The model under review builds one solid part; all positions refer to its coordinate system, in mm. Coordinates: 2 decimals unless noted, no trailing zeros. Write each loop counter-clockwise with the first axis right and the second up, starting at its lowest first coordinate (ties: lowest second). Pieces come first, ordered by that corner, then holes.
1) For line 1 (Y direction, x = 471, z = -1) (1 decimal); line 2 (Z direction, x = 927.5, y = -10), list the stretches that pass through material, from the lowest coordinate up.
2) For P1, Ø5, axis at y = 5.5, z = -2, coming from the +X side; P2, Ø24.5, axis at x = 553.5, y = 5, coming from the +Z side; P3, Ø24.5, axis at x = 596.5, y = -0.5, coming from the -Z side; P4, Ø14.5, axis at y = 5.5, z = 2, coming from the +X side, all flat-tipped, find the tip position at first contact; note any pin that passes through.
3) Add section B-B, the plane x = 849. State the section outline as (y, z) points (1 decimal).
from build123d import *

# Parameters (mm, degrees)
SKETCH1_W           = 28.575
SKETCH1_H           = 50.8
BOSS_EXTRUDE1_DEPTH = 1.5875
SKETCH1_3_W         = 1.5875
SKETCH1_3_H         = 50.8
BOSS_EXTRUDE2_DEPTH = 14.2875
SKETCH1_4_W         = 22.225
SKETCH1_4_H         = 22.225
SKETCH1_4_W_2       = 19.05
SKETCH1_4_H_2       = 19.05
BOSS_EXTRUDE3_DEPTH = 1016
BOSS_EXTRUDE4_DEPTH = 12.7
LPATTERN1_COUNT     = 2
LPATTERN1_PITCH     = 25.4


with BuildPart() as part:
    # Sketch1 → Boss-Extrude1 (new body)
    with BuildSketch(Plane(origin=(0, 0, 0), x_dir=(0, 0, -1), z_dir=(1, 0, 0))):
        Rectangle(SKETCH1_W, SKETCH1_H)
    extrude(amount=-BOSS_EXTRUDE1_DEPTH)

    # Sketch1<3> → Boss-Extrude2 (add)
    with BuildSketch(Plane(origin=(0, 0, 0), x_dir=(0, 0, -1), z_dir=(1, 0, 0))):
        with Locations((-13.49375, 0)):
            Rectangle(SKETCH1_3_W, SKETCH1_3_H)
        with Locations((13.49375, 0)):
            Rectangle(SKETCH1_3_W, SKETCH1_3_H)
    extrude(amount=-BOSS_EXTRUDE2_DEPTH)

    # Sketch1<4> → Boss-Extrude3 (add)
    with BuildSketch(Plane(origin=(0, 0, 0), x_dir=(0, 0, -1), z_dir=(1, 0, 0))):
        Rectangle(SKETCH1_4_W, SKETCH1_4_H)
        Rectangle(SKETCH1_4_W_2, SKETCH1_4_H_2, mode=Mode.SUBTRACT)
    extrude(amount=BOSS_EXTRUDE3_DEPTH)

    # 3DSketch1 → Boss-Extrude4 (add)
    with BuildSketch(Plane(origin=(-1.5875, 12.7, -6.35), x_dir=(0, 1, 0), z_dir=(0, 0, 1))):
        Polygon((0, 0), (0, 3.175), (6.35, 0), align=None)
    boss_extrude4 = extrude(amount=BOSS_EXTRUDE4_DEPTH)

    # LPattern1: Boss-Extrude4 ×2
    with Locations(*[(0, -i * LPATTERN1_PITCH, 0) for i in range(1, LPATTERN1_COUNT)]):
        add(boss_extrude4)


solid = part.part
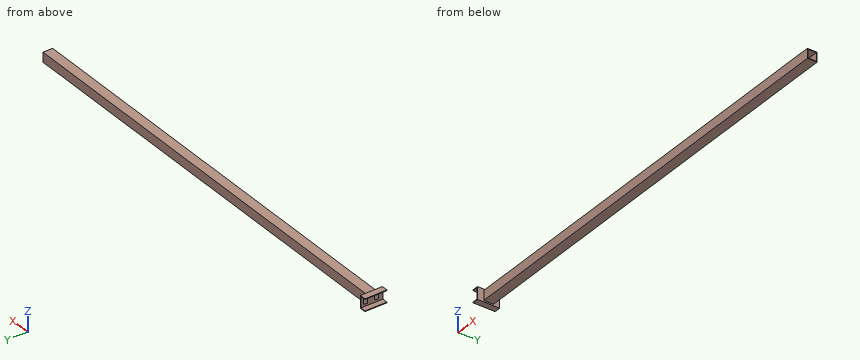
Geometry results:
1. line 1: y = -11.1 to -9.5, 9.5 to 11.1
1. line 2: z = -11.11 to 11.11
2. P1: stops at x = 0
2. P2: stops at z = 11.11
2. P3: stops at z = -11.11
2. P4: stops at x = 1016
3. outline: (-11.1, -11.1) - (11.1, -11.1) - (11.1, 11.1) - (-11.1, 11.1) - close; hole (-9.5, -9.5) - (9.5, -9.5) - (9.5, 9.5) - (-9.5, 9.5) - close
